CAD build for the part. Positions are in the model's coordinates, mm. A direction names the side the tool comes from. Round coordinates to 2 decimals unless told otherwise and drop trailing zeros.
from build123d import *

# Parameters (mm, degrees)
SKETCH1_W                                       = 15.875
SKETCH1_H                                       = 15.875
BOSS_EXTRUDE1_DEPTH                             = 497.84
SKETCH8_R                                       = 6.8199
CUT_EXTRUDE1_DEPTH                              = 13.08608
L_0_29_DIAMETER_HOLE1_D                         = 7.366
L_0_29_DIAMETER_HOLE1_DEPTH                     = 50.8
L_0_29_DIAMETER_HOLE1_TIP                       = 2.21296966
TAP_DRILL_FOR_6_32_TAP1_D                       = 2.7051
CBORE_FOR_10_SOCKET_HEAD_CAP_SCREW3_D           = 4.9784
CBORE_FOR_10_SOCKET_HEAD_CAP_SCREW3_DEPTH       = 25.4
CBORE_FOR_10_SOCKET_HEAD_CAP_SCREW3_CBORE_D     = 9.525
CBORE_FOR_10_SOCKET_HEAD_CAP_SCREW3_CBORE_DEPTH = 4.826
CBORE_FOR_10_SOCKET_HEAD_CAP_SCREW3_TIP         = 1.495662253
CBORE_FOR_10_SOCKET_HEAD_CAP_SCREW2_D           = 4.9784
CBORE_FOR_10_SOCKET_HEAD_CAP_SCREW2_DEPTH       = 25.4
CBORE_FOR_10_SOCKET_HEAD_CAP_SCREW2_CBORE_D     = 9.525
CBORE_FOR_10_SOCKET_HEAD_CAP_SCREW2_CBORE_DEPTH = 4.826
CBORE_FOR_10_SOCKET_HEAD_CAP_SCREW2_TIP         = 1.495662253
CBORE_FOR_10_SOCKET_HEAD_CAP_SCREW1_D           = 4.9784
CBORE_FOR_10_SOCKET_HEAD_CAP_SCREW1_DEPTH       = 25.4
CBORE_FOR_10_SOCKET_HEAD_CAP_SCREW1_CBORE_D     = 9.525
CBORE_FOR_10_SOCKET_HEAD_CAP_SCREW1_CBORE_DEPTH = 4.826
CBORE_FOR_10_SOCKET_HEAD_CAP_SCREW1_TIP         = 1.495662253


with BuildPart() as part:
    # Sketch1 → Boss-Extrude1 (new body)
    with BuildSketch(Plane.XY):
        with Locations((7.9375, 7.9375)):
            Rectangle(SKETCH1_W, SKETCH1_H)
    extrude(amount=BOSS_EXTRUDE1_DEPTH)

    # Sketch8 → Cut-Extrude1 (cut)
    with BuildSketch(Plane.ZY):
        with Locations((440.2201, 7.9375)):
            Circle(SKETCH8_R)
        with Locations((57.6199, 7.9375)):
            Circle(SKETCH8_R)
    extrude(amount=-CUT_EXTRUDE1_DEPTH, mode=Mode.SUBTRACT)

    # L (0.29) Diameter Hole1
    with Locations(Plane.ZY.offset(-13.08608)):
        with Locations((57.6199, 7.9375), (440.2201, 7.9375)):
            Hole(L_0_29_DIAMETER_HOLE1_D / 2, depth=L_0_29_DIAMETER_HOLE1_DEPTH)
            with Locations((0, 0, -(L_0_29_DIAMETER_HOLE1_DEPTH + L_0_29_DIAMETER_HOLE1_TIP / 2))):  # 118° drill point
                Cone(0, L_0_29_DIAMETER_HOLE1_D / 2, L_0_29_DIAMETER_HOLE1_TIP, mode=Mode.SUBTRACT)

    # Tap Drill for #6-32 Tap1 (through all)
    with Locations(Plane(origin=(-468.3125, 1840.244207037, -1707.973131805), x_dir=(0, 0, -1), z_dir=(-1, 0, 0))):
        with Locations((-2112.468131805, 1832.306707037), (-2080.718131805, 1832.306707037), (-2048.968131805, 1832.306707037), (-2017.218131805, 1832.306707037), (-1985.468131805, 1832.306707037), (-1953.718131805, 1832.306707037), (-1921.968131805, 1832.306707037), (-1890.218131805, 1832.306707037), (-1858.468131805, 1832.306707037), (-1826.718131805, 1832.306707037), (-1794.968131805, 1832.306707037)):
            Hole(TAP_DRILL_FOR_6_32_TAP1_D / 2)

    # CBORE for #10 Socket Head Cap Screw3
    with Locations(Plane(origin=(412.874136144, 0, -1707.973131805), x_dir=(-1, 0, 0), z_dir=(0, -1, 0))):
        with Locations((871.661636144, -2186.413131805), (871.661636144, -2199.813131805), (404.936636144, -2186.413131805), (404.936636144, -2199.813131805)):
            CounterBoreHole(CBORE_FOR_10_SOCKET_HEAD_CAP_SCREW3_D / 2, CBORE_FOR_10_SOCKET_HEAD_CAP_SCREW3_CBORE_D / 2, CBORE_FOR_10_SOCKET_HEAD_CAP_SCREW3_CBORE_DEPTH, depth=CBORE_FOR_10_SOCKET_HEAD_CAP_SCREW3_DEPTH)
            with Locations((0, 0, -(CBORE_FOR_10_SOCKET_HEAD_CAP_SCREW3_DEPTH + CBORE_FOR_10_SOCKET_HEAD_CAP_SCREW3_TIP / 2))):  # 118° drill point
                Cone(0, CBORE_FOR_10_SOCKET_HEAD_CAP_SCREW3_D / 2, CBORE_FOR_10_SOCKET_HEAD_CAP_SCREW3_TIP, mode=Mode.SUBTRACT)

    # CBORE for #10 Socket Head Cap Screw2
    with Locations(Plane(origin=(412.874136144, 15.875, -1707.973131805), x_dir=(1, 0, 0), z_dir=(0, 1, 0))):
        with Locations((-404.936636144, -1727.373131805), (-404.936636144, -1713.973131805), (-871.661636144, -1727.373131805), (-871.661636144, -1713.973131805)):
            CounterBoreHole(CBORE_FOR_10_SOCKET_HEAD_CAP_SCREW2_D / 2, CBORE_FOR_10_SOCKET_HEAD_CAP_SCREW2_CBORE_D / 2, CBORE_FOR_10_SOCKET_HEAD_CAP_SCREW2_CBORE_DEPTH, depth=CBORE_FOR_10_SOCKET_HEAD_CAP_SCREW2_DEPTH)
            with Locations((0, 0, -(CBORE_FOR_10_SOCKET_HEAD_CAP_SCREW2_DEPTH + CBORE_FOR_10_SOCKET_HEAD_CAP_SCREW2_TIP / 2))):  # 118° drill point
                Cone(0, CBORE_FOR_10_SOCKET_HEAD_CAP_SCREW2_D / 2, CBORE_FOR_10_SOCKET_HEAD_CAP_SCREW2_TIP, mode=Mode.SUBTRACT)

    # CBORE for #10 Socket Head Cap Screw1
    with Locations(Plane(origin=(15.875, 1702.05448625, -1707.973131805), x_dir=(0, 0, 1), z_dir=(1, 0, 0))):
        with Locations((2161.013131805, 1694.11698625), (2174.413131805, 1694.11698625)):
            CounterBoreHole(CBORE_FOR_10_SOCKET_HEAD_CAP_SCREW1_D / 2, CBORE_FOR_10_SOCKET_HEAD_CAP_SCREW1_CBORE_D / 2, CBORE_FOR_10_SOCKET_HEAD_CAP_SCREW1_CBORE_DEPTH, depth=CBORE_FOR_10_SOCKET_HEAD_CAP_SCREW1_DEPTH)
            with Locations((0, 0, -(CBORE_FOR_10_SOCKET_HEAD_CAP_SCREW1_DEPTH + CBORE_FOR_10_SOCKET_HEAD_CAP_SCREW1_TIP / 2))):  # 118° drill point
                Cone(0, CBORE_FOR_10_SOCKET_HEAD_CAP_SCREW1_D / 2, CBORE_FOR_10_SOCKET_HEAD_CAP_SCREW1_TIP, mode=Mode.SUBTRACT)


solid = part.part
Item 1: Mould opens along Z. For faces 1 (the cylindrical face through (8.97, 2.38, 496.49)), 2 (the flat face through (8, 15.875, 245)), 3 (the flat face through (8, 8, 497.84)) say: released by +Z, released by -Z, zero draft, split by the parting line, or undercut.
Verdict:
face 1: undercut
face 2: zero draft
face 3: released by +Z
Item 2: Cut at A-A (x = 8). State how many separate pieces and enclosed holes the cut face has, plus the area to 4 significant figures.
Verdict:
separate pieces: 5
enclosed holes: 15
area: 7,105 mm2
Item 3: Flat gauge pins, fed straight in: P1, Ø5.5, axis at y = 7.94, z = 466.44, coming from the +X side; P2, Ø3, axis at x = 8, z = 20.5, coming from the +Y side. Where does each tip first touch, or does it go through?
Verdict:
P1: stops at x = 11.05
P2: stops at y = 11.05
Item 4: Wall check: L1, parallel to Y at x = 3, z = 453.04 (3 decimals); L2, parallel to Z at x = 14, y = 9.75. Give the ranges that are in metal, low to high.
Verdict:
L1: y = 0 to 5.448, 10.427 to 15.875
L2: z = 0 to 54.41, 60.83 to 437.01, 443.43 to 448.64, 457.44 to 462.04, 470.84 to 497.84
Item 5: 3-axis set-ups, long thin cutter, end or side, ignore diameter. For faces 4 (the flat face through (11.049, 10, 455)), 5 (the flat face through (10, 11.049, 8)), 6 (the cylindrical face through (6.451, 9.986, 446.725)), 7 (the flat face through (6, 4.826, 494)): which of +Z, -Z, +X, -X, +Y, -Y reach the whole face in a straight line?
Verdict:
face 4: +X
face 5: +Y
face 6: -X
face 7: -Y
